Geometry: final body of the model. Coordinates: model frame, mm. Face numbers are marked on the shaded views. A direction names the side the tool comes from. Coordinates: 2 decimals unless noted, no trailing zeros. Write each loop counter-clockwise with the first axis right and the second up, starting at its lowest first coordinate (ties: lowest second). Pieces come first, ordered by that corner, then holes. Notation, with made-up numbers: (-24, -37.75) - (29, -37.75) arc R20 ccw to (29, -25.75) - close; hole circle Ø11 at (38.5, 30). An arc over 180 degrees is marked (long way). Answer as a JSON object with one key per item and string values. Group by question number.
Item 1: Line query: line 1 along Y through (x, z) = (143, -25); line 2 along Z through (x, y) = (-37.5, -269); line 3 along X through (y, z) = (-155, 4). Output: solid intervals per line, ascending. Write a range as from..to.
Item 2: Set-up query: the marked faces 1, 2 and 3. Return all of +Z, -Z, +X, -X, +Y, -Y with unobstructed straight access to the full face (end or side cutting, diameter ignored); none if empty.
Item 3: Mould query, pull axis X, two halves, no side actions, for the marked faces 4, 5 and 6. Classes: pulls with the +X half, pulls with the -X half, needs draft (parallel to the pull), parting line crosses it, or undercut.
Item 4: Section B-B on z = -174. Return loops of the section in (x, y).
Item 5: Section D-D on y = -130.5. Return loops of the section in (x, z), and give its area (3 significant figures).
Item 6: Section A-A on z = 100. Return loops of the section in (x, y), and give its area (3 significant figures).
Item 7: Section C-C on y = -479. Return loops of the section in (x, z), and give its area (3 significant figures).
Item 8: First-contact query: pin 1 Ø4 at (x, z) = (194.5, -109) entering from +Y; pin 2 Ø3 at (x, z) = (111, -37.5) entering from +Y; pin 3 Ø12 at (x, z) = (-87.64, -78.27) entering from -Y. Flat tips, straight axial feed; report the tip coordinate or a pass-through.
```python
from build123d import *

# Parameters (mm, degrees)
M30X2_0_1_D              = 28
M30X2_0_1_DEPTH          = 60
M30X2_0_1_TIP            = 8.412048666
CUT_EXTRUDE_1_REACH      = 651.173
SKETCH_4_R               = 35
PATTERN_CIRCULAR_1_COUNT = 3
SKETCH_5_R               = 5.25
CUT_EXTRUDE_2_DEPTH      = 30
PATTERN_CIRCULAR_2_COUNT = 3


with BuildPart() as part:
    # 草图1 → 旋转1 (revolve)
    with BuildSketch(Plane.XY, mode=Mode.PRIVATE) as revolve_1_sk:
        Polygon((0, 0), (-60, 0), (-60, -100), (-65, -100), (-65, -180), (-90, -205), (-90, -210), (-260, -210), (-260, -255), (-75, -255), (-75, -495), (-70, -495), (-70, -745), (0, -745), align=None)
    revolve(revolve_1_sk.sketch.rotate(Axis((0, -745, 0), (0, 1, 0)), 270), axis=Axis((0, -745, 0), (0, 1, 0)))

    # M30x2.0 螺纹孔1
    with Locations(Plane(origin=(0, 0, 0), x_dir=(1, 0, 0), z_dir=(0, 1, 0))):
        with Locations((0, 0)):
            Hole(M30X2_0_1_D / 2, depth=M30X2_0_1_DEPTH)
            with Locations((0, 0, -(M30X2_0_1_DEPTH + M30X2_0_1_TIP / 2))):  # 118° drill point
                Cone(0, M30X2_0_1_D / 2, M30X2_0_1_TIP, mode=Mode.SUBTRACT)

    # 草图4 → 切除-拉伸1 (cut, up to next)
    with BuildSketch(Plane(origin=(0, -210, 0), x_dir=(1, 0, 0), z_dir=(0, 1, 0)), mode=Mode.PRIVATE) as cut_extrude_1_sk1:
        with Locations(Location((-173.205080757, -100, 0), (0, 0, 270))):
            Circle(SKETCH_4_R)
    cut_extrude_1_tool1 = extrude(cut_extrude_1_sk1.sketch, amount=-CUT_EXTRUDE_1_REACH, mode=Mode.PRIVATE) & part.part
    cut_extrude_1 = cut_extrude_1_tool1.solids().sort_by_distance((-173.205081, -210, 100))[0]
    add(cut_extrude_1, mode=Mode.SUBTRACT)

    # 阵列(圆周)1: 切除-拉伸1 ×3 about axis
    pattern_circular_1_axis = Axis((0, 0, 0), (0, 1, 0))
    for i in range(1, PATTERN_CIRCULAR_1_COUNT):
        add(cut_extrude_1.rotate(pattern_circular_1_axis, i * 360 / PATTERN_CIRCULAR_1_COUNT), mode=Mode.SUBTRACT)

    # 草图5 → 切除-拉伸2 (cut)
    with BuildSketch(Plane(origin=(0, -210, 0), x_dir=(1, 0, 0), z_dir=(0, 1, 0))):
        with Locations(Location((-23.960098386, -115.031142241, 0), (0, 0, 270))):
            Circle(SKETCH_5_R)
        with Locations(Location((-104.106501212, -221.781055109, 0), (0, 0, 270))):
            Circle(SKETCH_5_R)
        with Locations(Location((-20.464389875, -244.143827993, 0), (0, 0, 270))):
            Circle(SKETCH_5_R)
    cut_extrude_2 = extrude(amount=-CUT_EXTRUDE_2_DEPTH, mode=Mode.SUBTRACT)

    # 阵列(圆周)2: 切除-拉伸2 ×3 about axis
    pattern_circular_2_axis = Axis((0, 0, 0), (0, 1, 0))
    for i in range(1, PATTERN_CIRCULAR_2_COUNT):
        add(cut_extrude_2.rotate(pattern_circular_2_axis, i * 360 / PATTERN_CIRCULAR_2_COUNT), mode=Mode.SUBTRACT)


solid = part.part
```
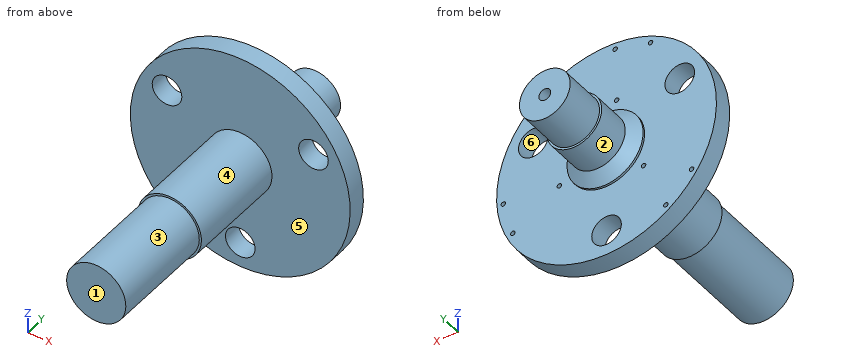
Checks:
{
 "1": {"line 1": "-255..-210", "line 2": "-64.95..64.95", "line 3": "-64.88..64.88"},
 "2": {"face 1": "+Z, -Z, +X, -X, -Y", "face 2": "+Y", "face 3": "-Y"},
 "3": {"face 4": "parting line crosses it", "face 5": "needs draft", "face 6": "undercut"},
 "4": {"outline": "(-193.19, -255) - (-23.43, -255) - (-23.43, -210) - (-193.19, -210) - close; (23.43, -255) - (193.19, -255) - (193.19, -210) - (23.43, -210) - close"},
 "5": {"outline": "circle Ø130 at (0, 0)", "area": "13,300 mm^2"},
 "6": {"outline": "(-240, -255) - (-208.21, -255) - (-208.21, -210) - (-240, -210) - close; (-138.21, -255) - (138.21, -255) - (138.21, -210) - (-138.21, -210) - close; (208.21, -255) - (240, -255) - (240, -210) - (208.21, -210) - close", "area": "15,300 mm^2"},
 "7": {"outline": "circle Ø150 at (0, 0)", "area": "17,700 mm^2"},
 "8": {"pin 1": "y = -210", "pin 2": "y = -240", "pin 3": "y = -255"}
}
